from build123d import *

# Parameters (mm, degrees)
F0_W     = 86.74343
F0_H     = 46.480264
F1_DEPTH = 25
F2_W     = 37.476842
F2_H     = 21.239644
F3_DEPTH = 63.6
F4_W     = 18.94737
F4_H     = 9.473686
F5_DEPTH = 25
F6_DEPTH = 25


with BuildPart() as f1:
    # F0 (on Front) → F1 (new body)
    with BuildSketch(Plane.XZ):
        Rectangle(F0_W, F0_H)
    extrude(amount=F1_DEPTH)

    # F2 (on Front) → F3 (join)
    with BuildSketch(Plane.XZ):
        Rectangle(F2_W, F2_H)
    extrude(amount=F3_DEPTH)

    # F4 (on Top) → F5 (join)
    with BuildSketch(Plane.XY):
        with Locations((-0.444079, -30.345397)):
            Rectangle(F4_W, F4_H)
    extrude(amount=-F5_DEPTH)

    # F4 (on Top) → F6 (join)
    with BuildSketch(Plane.XY):
        with Locations((-0.444079, -30.345397)):
            Rectangle(F4_W, F4_H)
    extrude(amount=F6_DEPTH)


solid = f1.part
Read the model definition and answer for the solid it produces. Units are mm, in the model's axes. A direction names the side the tool comes from. Round coordinates to 2 decimals unless told otherwise and drop trailing zeros. Write each loop counter-clockwise with the first axis right and the second up, starting at its lowest first coordinate (ties: lowest second). Pieces come first, ordered by that corner, then holes. Notation, with made-up numbers: M -37.5,44.5 L -28.5,44.5 A24 cw -28.5,80.5 Z; hole C -19,62 d3. An arc over 180 degrees is marked long. Use a Markdown table: item, result.
1) A tool of negligible diameter and unlimited length cuts with its end or side. For faces 1 (the flat face through (-18.738, -44, 0)), 2 (the flat face through (18.738, -44, 0)), 3 (the flat face through (-1, -25.609, 18)), 4 (the flat face through (-9.918, -30, -18)), 5 (the flat face through (9.03, -30, -18)), from which of +Z, -Z, +X, -X, +Y, -Y can it reach the whole face along a straight path? Write none if from no direction.
Answers follow:
| item | result |
|---|---|
| face 1 | +Z, -Z, -X, -Y |
| face 2 | +Z, -Z, +X, -Y |
| face 3 | +Z, +X, -X |
| face 4 | -Z, -X, -Y |
| face 5 | -Z, +X, -Y |
2) The part is cut by section C-C (x = 12.5). Write down the section's boundary in (y, z).
Answers follow:
| item | result |
|---|---|
| outline | M -63.6,-10.62 L -25,-10.62 L -25,-23.24 L 0,-23.24 L 0,23.24 L -25,23.24 L -25,10.62 L -63.6,10.62 Z |
3) The part is cut by section D-D (y = -58). Write down the section's boundary in (x, z).
Answers follow:
| item | result |
|---|---|
| outline | M -18.74,-10.62 L 18.74,-10.62 L 18.74,10.62 L -18.74,10.62 Z |
4) The part is cut by section B-B (z = 6.5). Write down the section's boundary in (x, y).
Answers follow:
| item | result |
|---|---|
| outline | M -43.37,-25 L -18.74,-25 L -18.74,-63.6 L 18.74,-63.6 L 18.74,-25 L 43.37,-25 L 43.37,0 L -43.37,0 Z |
5) Flat-ended cylindrical pins translate along their axes: pin 1 (1 mm diameter, centred on x = -31.5, z = 14.5, fed in from +Y); pin 2 (3 mm diameter, centred on y = -30.5, z = -17.5, fed in from +X); pin 3 (11 mm diameter, centred on x = 7.5, y = -53.5, fed in from +Z); pin 4 (3 mm diameter, centred on y = -31.5, z = 16.5, fed in from -X). Find the tip coordinate at first contact, or state that the pin passes through.
Answers follow:
| item | result |
|---|---|
| pin 1 | stops at y = 0 |
| pin 2 | stops at x = 9.03 |
| pin 3 | stops at z = 10.62 |
| pin 4 | stops at x = -9.92 |
6) The part is cut by section A-A (z = 15). Write down the section's boundary in (x, y).
Answers follow:
| item | result |
|---|---|
| outline | M -43.37,-25 L 43.37,-25 L 43.37,0 L -43.37,0 Z; M -9.92,-35.08 L 9.03,-35.08 L 9.03,-25.61 L -9.92,-25.61 Z |
7) Straight lines are drawn through the part: line 1 along Z through (x, y) = (-15, -55.5); line 2 along Z through (x, y) = (38, -18); line 3 along Y through (x, z) = (-20.5, 1). For each, find the intervals that lie inside material, in ascending order. Write a range as [from, to].
Answers follow:
| item | result |
|---|---|
| line 1 | z = [-10.62, 10.62] |
| line 2 | z = [-23.24, 23.24] |
| line 3 | y = [-25, 0] |
